Autodesk Inventor part; units mm, degrees
ref_plane "YZ Plane" through (0, 0, 0) normal (1, 0, 0) x (0, 1, 0)
ref_plane "XZ Plane" through (0, 0, 0) normal (0, 1, 0) x (-1, 0, 0)
ref_plane "XY Plane" through (0, 0, 0) normal (0, 0, 1) x (1, 0, 0)
sketch "Skizze1" plane through (0, 0, 0) normal (0, 0, 1) x (1, 0, 0)
  line L0 (-6, 12) -> (48, 12)
  line L1 (48, 12) -> (48, -12)
  line L2 (48, -12) -> (-6, -12)
  line L3 (-16.8, 0) -> (58.8, 0)
  line L4 (0, 16.8) -> (0, -16.8)
  line L5 (-6, 12) -> (-6, -12)
  point P0 (0, 0)
  dimension "d2" = 24
  dimension "d3" = 54
  dimension "d59" = 6
extrude "Extrusion1" add sketch "Skizze1" along normal blind 6
sketch "Skizze2" plane through (0, 0, 0) normal (0, 0, -1) x (-1, 0, 0)
  line L0 (-48, -12) -> (6, -12)
  line L1 (-48, 12) -> (-48, -12)
  line L2 (-48, 12) -> (6, 12)
  line L3 (6, -12) -> (-48, -12)
  line L4 (-48, -12) -> (-48, 12)
  line L5 (-48, 12) -> (6, 12)
  line L6 (6, 12) -> (6, -12)
  point P0 (0, 0)
extrude "Extrusion2" cut sketch "Skizze2" against normal blind 2
sketch "Skizze3" plane through (0, 0, 2) normal (0, 0, -1) x (-1, 0, 0)
  line L0 (6, -12) -> (-48, -12)
  line L1 (-48, -12) -> (-48, 12)
  line L2 (-48, 12) -> (6, 12)
  line L3 (-48, -12) -> (-44, -12)
  line L4 (-44, -12) -> (-44, 12)
  line L5 (-44, 12) -> (-48, 12)
  line L6 (-48, 12) -> (-48, -12)
  point P0 (0, 0)
  point P1 (0, -12.5)
  dimension "d9" = 4
extrude "Extrusion3" [suppressed]
sketch "Skizze4" plane through (0, 0, 6) normal (0, 0, 1) x (1, 0, 0)
  line L0 (48, -12) -> (48, 12)
  line L1 (-17, 0) -> (60, 0)
  point P0 (0, 0)
  point P1 (46, 0)
  dimension "d12" = 2
hole "Bohrung1" [suppressed]
pattern_linear "Rechteckige Anordnung1" [suppressed]
sketch "Skizze7" plane through (0, 0, 2) normal (0, 0, -1) x (-1, 0, 0)
  line L0 (6, -12) -> (-48, -12)
  line L1 (6, 12) -> (6, -12)
  line L2 (-48, 12) -> (6, 12)
  line L3 (-48, 12) -> (6, 12)
  line L4 (6, -12) -> (0, -12)
  line L5 (0, -12) -> (0, 12)
  line L6 (0, 12) -> (6, 12)
  line L7 (6, 12) -> (6, -12)
  line L8 (-48, -12) -> (-48, 12)
  point P0 (0, 0)
  point P1 (-44, 12)
extrude "Extrusion4" add sketch "Skizze7" along normal blind 2.8 contours L0 L5 L2 L1
sketch "Skizze8" plane through (0, 0, -0.8) normal (0, 0, -1) x (-1, 0, 0)
  line L0 (6, -12) -> (6, 12)
  line L1 (6, 12) -> (0, 12)
  line L2 (0, 12) -> (0, -12)
  line L3 (0, -12) -> (6, -12)
  line L4 (-58.8, 0) -> (16.8, 0)
  line L5 (6, 12) -> (0, 12)
  line L6 (0, 12) -> (0, 24)
  line L7 (0, 24) -> (6, 24)
  line L8 (6, 24) -> (6, 12)
  line L9 (6, -12) -> (-48, -12)
  line L10 (6, -12) -> (0, -12)
  line L11 (0, -12) -> (0, -24)
  line L12 (0, -24) -> (6, -24)
  line L13 (6, -24) -> (6, -12)
  line L14 (6, -12) -> (6, 12)
  dimension "d67" = 48
extrude "Extrusion5" add sketch "Skizze8" against normal up to surface (6.8 mm away)
sketch "Skizze9" plane through (0, 0, 6) normal (0, 0, 1) x (1, 0, 0)
  line L0 (0, -12) -> (48, -12)
  line L1 (48, -12) -> (48, 12)
  line L2 (48, 12) -> (0, 12)
  line L3 (0, 24) -> (0, 12)
  line L4 (-6, 24) -> (0, 24)
  line L5 (-6, -24) -> (-6, 24)
  line L6 (0, -24) -> (-6, -24)
  line L7 (0, -12) -> (0, -24)
  line L8 (48, 12) -> (0, 12)
  arc A0 (0, 12) -> (3.6, 12) centre (1.8, 12) ccw
  line L9 (0, -12) -> (48, -12)
  arc A1 (3.6, -12) -> (0, -12) centre (1.8, -12) ccw
  line L10 (-16.8, 0) -> (58.8, 0)
  point P0 (0, 0)
  point P1 (44, 12)
  point P2 (44, -12)
  dimension "d68" = 1.8
extrude "Extrusion6" cut sketch "Skizze9" against normal through all contours A1 L0 | A0 L2
fillet "Rundung1" radius 2 4 edges at (0, -12, 4) (3.6, -12, 4) (0, 12, 4) (3.6, 12, 4)
sketch "Skizze10" plane through (0, 0, -0.8) normal (0, 0, -1) x (-1, 0, 0)
  line L0 (0, -24) -> (0, 24)
  line L1 (-58.8, 0) -> (16.8, 0)
  line L2 (0, -22) -> (6, -22) construction
  line L3 (6, 24) -> (6, -24)
  point P0 (0, 0)
  point P1 (3, -22)
  point P2 (3, 22)
  dimension "d72" = 22
hole "Bohrung4" at (-3, -22, -0.8) at (-3, 22, -0.8) direction (0, 0, 1) diameter 1.567 end through all
fillet "Rundung2" radius 1 4 edges at (0, 24, 2.6) (-6, 24, 2.6) (0, -24, 2.6) (-6, -24, 2.6)
sketch "Skizze11" plane through (0, 0, -0.8) normal (0, 0, -1) x (-1, 0, 0)
  arc A0 (5, -24) -> (6, -23) centre (5, -23) ccw
  line L0 (6, 23) -> (6, -23)
  arc A1 (6, 23) -> (5, 24) centre (5, 23) ccw
  line L1 (1, 24) -> (5, 24)
  arc A2 (1, 24) -> (0, 23) centre (1, 23) ccw
  line L2 (0, -23) -> (0, 23)
  arc A3 (0, -23) -> (1, -24) centre (1, -23) ccw
  line L3 (5, -24) -> (1, -24)
  circle A4 centre (3, -22) radius 0.7835
  circle A5 centre (3, 22) radius 0.7835
  point P0 (0, 0)
extrude "Extrusion7" cut sketch "Skizze11" against normal blind 0.2
sketch "Skizze12" plane through (0, 0, 6) normal (0, 0, 1) x (1, 0, 0)
  line L0 (48, -12) -> (48, 12) construction
  line L1 (-16.8, 0) -> (58.8, 0) construction
  line L2 (48, -12) -> (48, 12)
  line L3 (48, 8) -> (42, 8)
  line L4 (40, 6) -> (40, -6)
  line L5 (42, -8) -> (48, -8)
  line L6 (48, -8) -> (48, 8)
  arc A0 (42, 8) -> (40, 6) centre (42, 6) ccw
  arc A1 (40, -6) -> (42, -8) centre (42, -6) ccw
  point P0 (0, 0)
  dimension "d83" = 2
  dimension "d84" = 4
  dimension "d85" = 8
extrude "Extrusion8" cut sketch "Skizze12" against normal blind 2
sketch "Skizze13" plane through (0, 0, 2) normal (0, 0, -1) x (-1, 0, 0)
  line L0 (-48, -12) -> (-48, 12) construction
  line L1 (-58.8, 0) -> (16.8, 0) construction
  line L2 (-48, -7.9) -> (-53.8, -7.9)
  line L3 (-55.8, -5.9) -> (-55.8, 5.9)
  line L4 (-53.8, 7.9) -> (-48, 7.9)
  line L5 (-48, 7.9) -> (-48, -7.9)
  arc A0 (-55.8, -5.9) -> (-53.8, -7.9) centre (-53.8, -5.9) ccw
  arc A1 (-53.8, 7.9) -> (-55.8, 5.9) centre (-53.8, 5.9) ccw
  point P0 (0, 0)
  dimension "d88" = 2
  dimension "d89" = 4.1
  dimension "d90" = 7.8
extrude "Extrusion9" add sketch "Skizze13" against normal blind 2
sketch "Skizze14" plane through (0, 0, 2) normal (0, 0, -1) x (-1, 0, 0)
  line L0 (-48, -12) -> (-48, -7.9) construction
  line L1 (-68.16, 0) -> (18.36, 0) construction
  line L2 (-44, -4) -> (-52, -4) construction
  line L3 (-52, -4) -> (-52, 4) construction
  line L4 (-52, 4) -> (-44, 4) construction
  line L5 (-44, 4) -> (-44, -4) construction
  point P0 (0, 0)
  dimension "d93" = 8
  dimension "d94" = 8
hole "Bohrung5" at (44, -4, 2) at (52, -4, 2) at (52, 4, 2) at (44, 4, 2) direction (0, 0, 1) diameter 3 end through all countersink diameter 6.7 countersink angle 90
fillet "Rundung3" radius 2 4 edges at (48, -8, 5) (48, -7.9, 3) (48, 8, 5) (48, 7.9, 3)
properties part number "Kicker Chip" material "Aluminium 6061"
Geometry check sheet. Reference: the model listing, model coordinates, mm. A direction names the side the tool comes from. Give positions to 0.01 mm unless a question says otherwise; leave off trailing zeros. Loops run counter-clockwise (first coordinate to the right, second up) from the corner with the lowest first, then second, coordinate; pieces in that order, holes last. Notation, with made-up numbers: M 33.25,59.25 L 47.25,59.25 A19 cw 47.25,70.25 Z; hole C 52,85 d2. An arc over 180 degrees is marked long. Answer as a JSON object with one key per item and string values. Group by question number.
Item 1: Material ranges on L1, parallel to Y at x = 44, z = 3.9; L2, parallel to X at y = -4, z = 3.9; L3, parallel to Y at x = 52, z = 3.95, recorded low to high.
Item 2: Sectioned sample at B-B on y = -4. Record the boundary of the cut face in (x, z), plus the area to 3 significant figures.
Item 3: Sectioned sample at D-D on x = 44. Record the boundary of the cut face in (y, z), plus the area to 3 significant figures.
Item 4: Sectioned sample at A-A on x = -3. Record the boundary of the cut face in (y, z), plus the area to 3 significant figures.
Item 5: Mould release check, pull along Y, two halves, no side actions. Record for faces 6 (the cylindrical face through (47.43, 8.6, 4.99)), 7 (the flat face through (48, 11, 4)), 8 (the flat face through (-3, -24, 3)): pulls with the +Y half, pulls with the -Y half, needs draft (parallel to the pull), parting line crosses it, or undercut.
Item 6: Access from +Z, -Z, +X, -X, +Y, -Y to the whole of each face (thin tool, end or side, straight path). Record for faces 1 (the flat face through (52, 7.9, 3)), 2 (the flat face through (22, 0, 2)), 3 (the cylindrical face through (4.07, -11.754, 3.972)), 4 (the cylindrical face through (40.6, 7.43, 5.01)), 5 (the flat face through (52, -7.9, 3)).
Item 7: Sectioned sample at C-C on y = -22. Record the boundary of the cut face in (x, z).
Item 8: Gauge pin test, flat ends, axial feed: pin 1 (1 mm diameter, centred on x = 52.5, z = 3, fed in from +Y); pin 2 (0.6 mm diameter, centred on y = 11, z = 4, fed in from +X); pin 3 (3 mm diameter, centred on x = 19, z = 4, fed in from +Y). Record the tip position at first contact, or that the pin passes through.
Findings below:
{
 "1": {"L1": "-12 to -5.5, -2.5 to 2.5, 5.5 to 12", "L2": "-6 to 42.5, 45.5 to 50.5, 53.5 to 55.8", "L3": "-7.9 to -5.5, -2.5 to 2.5, 5.5 to 7.9"},
 "2": {"outline": "M -6,-0.6 L 0,-0.6 L 0,2 L 40.65,2 L 42.5,3.85 L 42.5,4 L 40,4 L 40,6 L -6,6 Z; M 45.5,3.85 L 47.35,2 L 48.65,2 L 50.5,3.85 L 50.5,4 L 45.5,4 Z; M 53.5,3.85 L 55.35,2 L 55.8,2 L 55.8,4 L 53.5,4 Z", "area": "212 mm2"},
 "3": {"outline": "M -12,2 L -7.35,2 L -5.5,3.85 L -5.5,4 L -8,4 L -8,6 L -12,6 Z; M -2.5,3.85 L -0.65,2 L 0.65,2 L 2.5,3.85 L 2.5,4 L -2.5,4 Z; M 5.5,3.85 L 7.35,2 L 12,2 L 12,6 L 8,6 L 8,4 L 5.5,4 Z", "area": "45.2 mm2"},
 "4": {"outline": "M -24,-0.6 L -22.78,-0.6 L -22.78,6 L -24,6 Z; M -21.22,-0.6 L 21.22,-0.6 L 21.22,6 L -21.22,6 Z; M 22.78,-0.6 L 24,-0.6 L 24,6 L 22.78,6 Z", "area": "296 mm2"},
 "5": {"face 6": "undercut", "face 7": "needs draft", "face 8": "pulls with the -Y half"},
 "6": {"face 1": "+Z, -Z, +X, +Y", "face 2": "-Z, +X, +Y, -Y", "face 3": "+Z, -Z, -Y", "face 4": "+Z, +X", "face 5": "+Z, -Z, +X, -Y"},
 "7": {"outline": "M -6,-0.6 L -3.78,-0.6 L -3.78,6 L -6,6 Z; M -2.22,-0.6 L 0,-0.6 L 0,6 L -2.22,6 Z"},
 "8": {"pin 1": "y = 7.9", "pin 2": "x = 48", "pin 3": "y = 12"}
}
